```python
from build123d import *

# Parameters (mm, degrees)
BOSS_EXTRUDE2_DEPTH             = 76.2
BOSS_EXTRUDE3_DEPTH             = 118.4125
SKETCH5_W                       = 96.825174549
SKETCH5_H                       = 1.5875
CUT_EXTRUDE2_DEPTH              = 76.2
BOSS_EXTRUDE5_REACH             = 52
BOSS_EXTRUDE5_DIRECTION_2_REACH = 52
BOSS_EXTRUDE6_REACH             = 122.202
BOSS_EXTRUDE7_DEPTH             = 1.5875
BOSS_EXTRUDE8_DEPTH             = 1.5875
SKETCH15_W                      = 143.32634152
SKETCH15_H                      = 53.255725939
CUT_EXTRUDE3_DEPTH              = 264.5875
CUT_EXTRUDE4_DEPTH              = 264.5875
SKETCH18_R                      = 2.5
CUT_EXTRUDE5_DEPTH              = 264.5875


with BuildPart() as part:
    # Sketch1 → Boss-Extrude2 (new body)
    with BuildSketch(Plane(origin=(0, 0, 0), x_dir=(1, 0, 0), z_dir=(0, 1, 0))):
        Polygon((1.5875, -1.5875), (98.4125, -1.5875), (98.4125, -118.4125), (98.4125, -120), (100, -120), (100, 0), (0, 0), (0, -120), (1.5875, -120), (1.5875, -118.4125), align=None)
    extrude(amount=BOSS_EXTRUDE2_DEPTH)

    # Sketch2 → Boss-Extrude3 (add)
    with BuildSketch(Plane.XY.offset(120)):
        Polygon((0, 0), (1.5875, 0.917396042), (50, -26.981614962), (98.4125, 0.917396042), (100, 0), (50, -28.813850766), align=None)
    extrude(amount=-BOSS_EXTRUDE3_DEPTH)

    # Sketch5 → Cut-Extrude2 (cut)
    with BuildSketch(Plane(origin=(0, 76.2, 0), x_dir=(1, 0, 0), z_dir=(0, 1, 0))):
        with Locations((49.999912726, -0.79375)):
            Rectangle(SKETCH5_W, SKETCH5_H)
    extrude(amount=-CUT_EXTRUDE2_DEPTH, mode=Mode.SUBTRACT)

    # Boss-Extrude5: up to this face of the body (flat: up to its plane)
    boss_extrude5_end = Plane(part.part.faces().sort_by_distance((0, 38.1, 60))[0])
    # Sketch11 → Boss-Extrude5 (add, up to the picked face)
    with BuildSketch(Plane.ZY.offset(-50), mode=Mode.PRIVATE) as boss_extrude5_sk1:
        Polygon((1.5875, -26.981614962), (1.5875, -28.813850766), (-27.384499219, 0), (-25.76142568, 0), align=None)
    boss_extrude5_tool1 = split(extrude(boss_extrude5_sk1.sketch, amount=BOSS_EXTRUDE5_REACH, mode=Mode.PRIVATE), bisect_by=boss_extrude5_end, keep=Keep.BOTH, mode=Mode.PRIVATE)
    add(boss_extrude5_tool1.solids().sort_by_distance((50, -14.256717, -12.190864))[0])
    # Sketch11 → Boss-Extrude5 (add, up to the picked face)
    with BuildSketch(Plane.ZY.offset(-50), mode=Mode.PRIVATE) as boss_extrude5_sk2:
        Polygon((-27.384499219, 0), (-25.76142568, 0), (-117.814066128, 90.816324189), (-118.614630338, 90.004861602), align=None)
    boss_extrude5_tool2 = split(extrude(boss_extrude5_sk2.sketch, amount=BOSS_EXTRUDE5_REACH, mode=Mode.PRIVATE), bisect_by=boss_extrude5_end, keep=Keep.BOTH, mode=Mode.PRIVATE)
    add(boss_extrude5_tool2.solids().sort_by_distance((50, 45.2056, -72.392749))[0])

    # Boss-Extrude5 direction 2: up to this face of the body (flat: up to its plane)
    boss_extrude5_direction_2_end = Plane(part.part.faces().sort_by_distance((100, 38.1, 60))[0])
    # Sketch11 → Boss-Extrude5 direction 2 (add, up to the picked face)
    with BuildSketch(Plane.ZY.offset(-50), mode=Mode.PRIVATE) as boss_extrude5_direction_2_sk1:
        Polygon((1.5875, -26.981614962), (1.5875, -28.813850766), (-27.384499219, 0), (-25.76142568, 0), align=None)
    boss_extrude5_direction_2_tool1 = split(extrude(boss_extrude5_direction_2_sk1.sketch, amount=-BOSS_EXTRUDE5_DIRECTION_2_REACH, mode=Mode.PRIVATE), bisect_by=boss_extrude5_direction_2_end, keep=Keep.BOTH, mode=Mode.PRIVATE)
    add(boss_extrude5_direction_2_tool1.solids().sort_by_distance((50, -14.256717, -12.190864))[0])
    # Sketch11 → Boss-Extrude5 direction 2 (add, up to the picked face)
    with BuildSketch(Plane.ZY.offset(-50), mode=Mode.PRIVATE) as boss_extrude5_direction_2_sk2:
        Polygon((-27.384499219, 0), (-25.76142568, 0), (-117.814066128, 90.816324189), (-118.614630338, 90.004861602), align=None)
    boss_extrude5_direction_2_tool2 = split(extrude(boss_extrude5_direction_2_sk2.sketch, amount=-BOSS_EXTRUDE5_DIRECTION_2_REACH, mode=Mode.PRIVATE), bisect_by=boss_extrude5_direction_2_end, keep=Keep.BOTH, mode=Mode.PRIVATE)
    add(boss_extrude5_direction_2_tool2.solids().sort_by_distance((50, 45.2056, -72.392749))[0])

    # Boss-Extrude6: up to this face of the body (flat: up to its plane)
    boss_extrude6_end = Plane(part.part.faces().sort_by_distance((50, -14.406925383, -12.89849961))[0])
    # Sketch12 → Boss-Extrude6 (add, up to the picked face)
    with BuildSketch(Plane(origin=(0, 0, 1.5875), x_dir=(-1, 0, 0), z_dir=(0, 0, -1)), mode=Mode.PRIVATE) as boss_extrude6_sk1:
        Polygon((-50, -26.981614962), (-98.4125, 0.917396042), (-98.4125, 0), (-100, 0), (-53.179435853, -26.981614962), (-50, -28.813850766), (-46.820564147, -26.981614962), (0, 0), (0, 0.917396042), (-1.5875, 0.917396042), align=None)
    boss_extrude6_tool1 = split(extrude(boss_extrude6_sk1.sketch, amount=BOSS_EXTRUDE6_REACH, mode=Mode.PRIVATE), bisect_by=boss_extrude6_end, keep=Keep.BOTH, mode=Mode.PRIVATE)
    add(boss_extrude6_tool1.solids().sort_by_distance((25.272847, -13.93602, 1.5875))[0])

    # Sketch13 → Boss-Extrude7 (add)
    with BuildSketch(Plane.ZY):
        Polygon((0, 0.917396042), (0, 76.2), (-102.998764504, 76.2), (-26.691310574, 0.917396042), align=None)
    extrude(amount=-BOSS_EXTRUDE7_DEPTH)

    # Sketch14 → Boss-Extrude8 (add)
    with BuildSketch(Plane(origin=(100, 0, 0), x_dir=(0, 0, -1), z_dir=(1, 0, 0))):
        Polygon((0, 0), (25.76142568, 0), (102.998764504, 76.2), (0, 76.2), align=None)
    extrude(amount=-BOSS_EXTRUDE8_DEPTH)

    # Sketch15 → Cut-Extrude3 (cut)
    with BuildSketch(Plane.XY.offset(120)):
        with Locations((28.33682924, 102.82786297)):
            Rectangle(SKETCH15_W, SKETCH15_H)
    extrude(amount=-CUT_EXTRUDE3_DEPTH, mode=Mode.SUBTRACT)

    # Sketch16 → Cut-Extrude4 (cut)
    with BuildSketch(Plane.XY.offset(120)):
        Polygon((63.760723445, -52.692511686), (50, -28.813850766), (100, 0), (131.48806996, 0), (150.508378032, -66.092213095), align=None)
        Polygon((-24.631729482, 0), (0, 0), (50, -28.813850766), (-14.891819722, -42.472870615), align=None)
    extrude(amount=-CUT_EXTRUDE4_DEPTH, mode=Mode.SUBTRACT)

    # Sketch18 → Cut-Extrude5 (cut)
    with BuildSketch(Plane.ZY):
        with Locations((106.931013832, 67.039572628)):
            Circle(SKETCH18_R)
    extrude(amount=-CUT_EXTRUDE5_DEPTH, mode=Mode.SUBTRACT)


solid = part.part
```
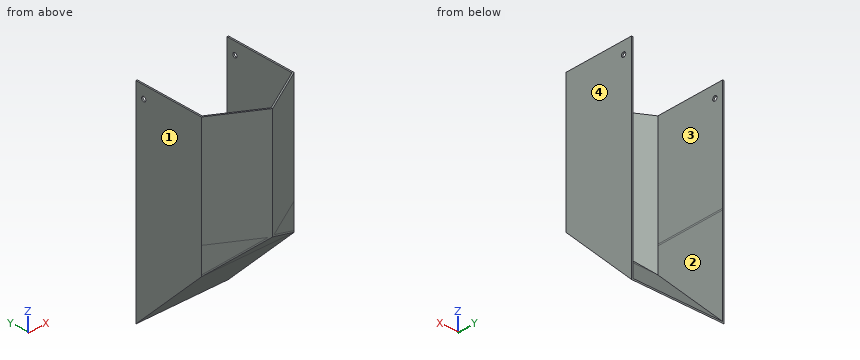
Read the model definition and answer for the solid it produces. Units are mm, in the model's axes. Face numbers are marked on the shaded views. Coordinates: 2 decimals unless noted, no trailing zeros. Write each loop counter-clockwise with the first axis right and the second up, starting at its lowest first coordinate (ties: lowest second). Pieces come first, ordered by that corner, then holes. Notation, with made-up numbers: (19, 85.5) - (78, 85.5) arc R19 cw to (78, 89.5) - close; hole circle Ø4 at (24.5, 56.25). An arc over 180 degrees is marked (long way). Answer as a JSON object with one key per item and string values. Group by question number.
1. A cutting plane is placed at D-D (z = -83). Determine the outline of the cut face in (x, y), plus the area to 3 significant figures.
2. A cutting plane is placed at A-A (z = 19). Determine the outline of the cut face in (x, y), plus the area to 3 significant figures.
3. A cutting plane is placed at B-B (x = 35). Determine the outline of the cut face in (y, z), plus the area to 3 significant figures.
4. The mould has two halves that part along X. Classify the marked faces 1, 2, 3 and 4: +X half, -X half, draft (parallel to the pull), parting line (faces both ways), or undercut.
5. Consider L1, parallel to X at y = 36, z = -14; L2, parallel to X at y = -9, z = 98.5; L3, parallel to Z at x = 86, y = 0.5. Determine where each line is inside the solid, lowest interval first. Write a range as [from, to].
6. A cutting plane is placed at C-C (y = -14). Determine the outline of the cut face in (x, z).
7. Each of these flat-tipped pins is pushed along its axis until it touches: P1, Ø6.5, axis at y = 67.04, z = 106.93, coming from the -X side; P2, Ø1.5, axis at x = 40, z = 53, coming from the -Y side; P3, Ø5, axis at x = 40.5, y = 55, coming from the +Z side; P4, Ø12, axis at x = 39, z = 49.5, coming from the +Y side. Where does it stop, or does it pass through?
Worked out:
{
 "1": {"outline": "(0, 54.87) - (100, 54.87) - (100, 76.2) - (98.41, 76.2) - (98.41, 56.47) - (1.59, 56.47) - (1.59, 76.2) - (0, 76.2) - close", "area": "223 mm²"},
 "2": {"outline": "(0, 0) - (50, -28.81) - (100, 0) - (100, 76.2) - (98.41, 76.2) - (98.41, 0.92) - (50, -26.98) - (1.59, 0.92) - (1.59, 76.2) - (0, 76.2) - close", "area": "421 mm²"},
 "3": {"outline": "(-20.17, -7.1) - (0, -27.38) - (76.2, -104.62) - (76.2, -103) - (-18.34, -7.17) - (-18.34, 120) - (-20.17, 120) - close", "area": "389 mm²"},
 "4": {"face 1": "-X half", "face 2": "undercut", "face 3": "undercut", "face 4": "+X half"},
 "5": {"L1": "x = [0, 1.59], [98.41, 100]", "L2": "x = [15.62, 18.8], [81.2, 84.38]", "L3": "z = [-27.89, -26.27]"},
 "6": {"outline": "(24.29, -13.31) - (75.71, -13.31) - (75.71, 120) - (72.53, 120) - (72.53, -11.57) - (27.47, -11.57) - (27.47, 120) - (24.29, 120) - close"},
 "7": {"P1": "stops at x = 0", "P2": "stops at y = -23.48", "P3": "stops at z = -78.98", "P4": "stops at y = -17.18"}
}
